Job drawing, mm, ordinate dimensions from the low corner. One solid piece. A direction names the side the tool comes from. Round coordinates to 2 decimals unless told otherwise and drop trailing zeros. Loops run counter-clockwise (first coordinate to the right, second up) from the corner with the lowest first, then second, coordinate; pieces in that order, holes last. Notation, with made-up numbers: M 21.5,-19.75 L 25.5,-19.75 A33 ccw 25.5,17.25 Z; hole C 73.25,62.5 d5. An arc over 180 degrees is marked long. Write each question's results on one line, items separated by ' | '. Start each with the question number.
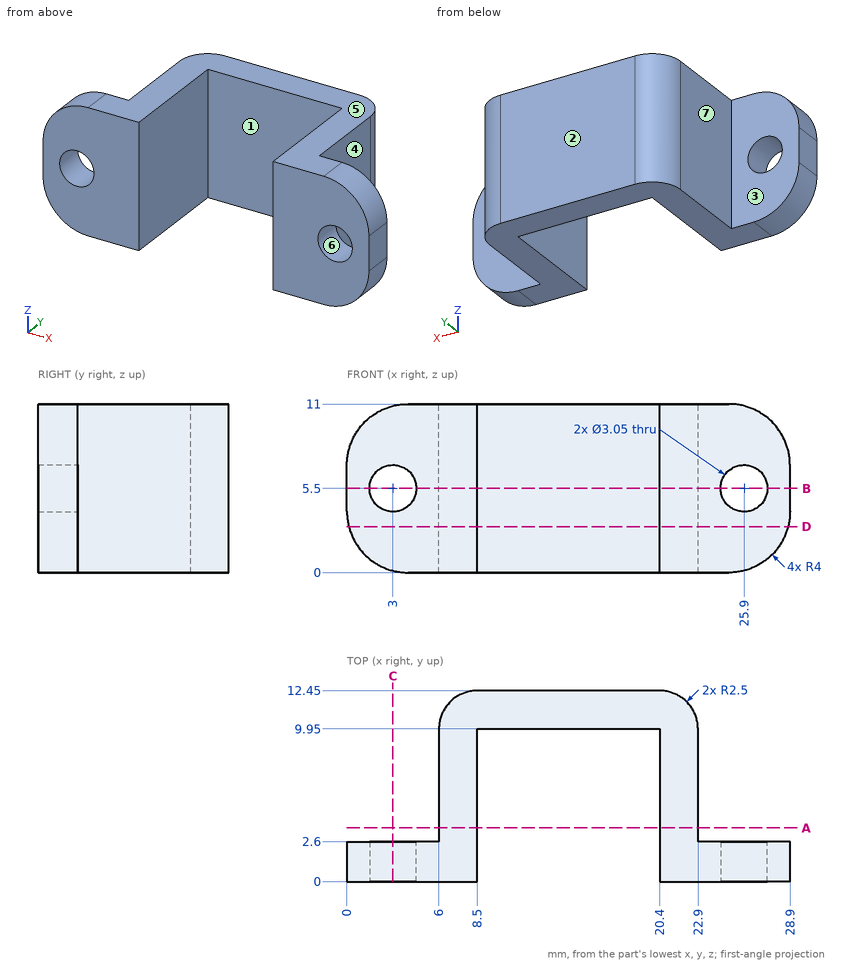
Item 1: Drill centre lines: line 1 along X through (y, z) = (9.5, 4.5); line 2 along Y through (x, z) = (25.5, 1.5); line 3 along Y through (x, z) = (18.5, 1). Where is each one in solid material? Low to high. Write a range as [from, to].
Item 2: Saw through at C-C, the plane x = 3. Give the cut face in (y, z) (3 decimals).
Item 3: Saw through at D-D, the plane z = 3. Give the cut face in (x, y).
Item 4: Mould opens along Z. For the marked faces 5, 6 and 7 say: released by +Z, released by -Z, zero draft, split by the parting line, or undercut.
Item 5: Saw through at B-B, the plane z = 5.5. Give the cut face in (x, y) (3 decimals), then the cut area to 3 significant figures.
Item 6: Saw through at A-A, the plane y = 3.5. Give the cut face in (x, z).
Item 7: Tool access for the marked faces 1, 2, 3 and 4: list every direction of +Z, -Z, +X, -X, +Y, -Y with a clear straight run to the whole face (end or side of a thin tool).
Item 8: Drop flat-ended pins along their axis: pin 1 (3.5 mm diameter, centred on y = 4.5, z = 5.5, fed in from +X); pin 2 (3 mm diameter, centred on y = 4, z = 3, fed in from -X); pin 3 (5 mm diameter, centred on x = 26.5, z = 4.5, fed in from +Y); pin 4 (2.5 mm diameter, centred on x = 3, z = 5.5, fed in from +Y). Give the stop position or say it passes through.
Working result:
1) line 1: x = [6, 8.5], [20.4, 22.9] | line 2: y = [0, 2.6] | line 3: y = [9.95, 12.45]
2) outline: M 0,0.127 L 2.6,0.127 L 2.6,3.975 L 0,3.975 Z; M 0,7.025 L 2.6,7.025 L 2.6,10.873 L 0,10.873 Z
3) outline: M 0.13,0 L 8.5,0 L 8.5,9.95 L 20.4,9.95 L 20.4,0 L 28.77,0 L 28.77,2.6 L 22.9,2.6 L 22.9,9.95 A2.5 ccw 20.4,12.45 L 8.5,12.45 A2.5 ccw 6,9.95 L 6,2.6 L 0.13,2.6 Z
4) face 5: released by +Z | face 6: undercut | face 7: zero draft
5) outline: M 0,0 L 1.475,0 L 1.475,2.6 L 0,2.6 Z; M 4.525,0 L 8.5,0 L 8.5,9.95 L 20.4,9.95 L 20.4,0 L 24.375,0 L 24.375,2.6 L 22.9,2.6 L 22.9,9.95 A2.5 ccw 20.4,12.45 L 8.5,12.45 A2.5 ccw 6,9.95 L 6,2.6 L 4.525,2.6 Z; M 27.425,0 L 28.9,0 L 28.9,2.6 L 27.425,2.6 Z | area: 105 mm²
6) outline: M 6,0 L 8.5,0 L 8.5,11 L 6,11 Z; M 20.4,0 L 22.9,0 L 22.9,11 L 20.4,11 Z
7) face 1: +Z, -Z, -Y | face 2: +Z, -Z, +X, -X, +Y | face 3: +Z, -Z, -X, +Y | face 4: +Z, -Z, +X, +Y
8) pin 1: stops at x = 22.9 | pin 2: stops at x = 0.03 | pin 3: stops at y = 2.6 | pin 4: passes through
